Check sheet for the modelled part. Datum: model origin and axes. Units: mm. Face numbers are marked on the shaded views. A direction names the side the tool comes from. Round coordinates to 2 decimals unless told otherwise and drop trailing zeros. Loops run counter-clockwise (first coordinate to the right, second up) from the corner with the lowest first, then second, coordinate; pieces in that order, holes last. Notation, with made-up numbers: (63, -23) - (122, -23) arc R17 ccw to (122, 8) - close; hole circle Ø7 at (54.5, -32). An arc over 180 degrees is marked (long way). Put each result on its own line as item: value. Start each with the question number.
Item 1: Gauge pin test, flat ends, axial feed: pin 1 Ø8 at (x, y) = (-4, -1) entering from +Z; pin 2 Ø1 at (x, y) = (8, -2.5) entering from -Z. Record the tip position at first contact, or that the pin passes through.
Item 2: Draft check along Y on the marked faces 4, 5 and 6. Enter one of: pulls with the +Y half, pulls with the -Y half, needs draft (parallel to the pull), parting line crosses it, or undercut.
Item 3: Section check C-C, the plane z = 6.5. Record the cut outline in (x, y).
Item 4: Section check D-D, the plane y = 6. Record the cut outline in (x, z), and give its area (3 significant figures).
Item 5: Tool access check on the marked faces 1, 2 and 3. Record the directions out of +Z, -Z, +X, -X, +Y, -Y that give a thin tool (end or side, any length) a straight path to the whole face; none if there is none.
Item 6: Material ranges on line 1 along X through (y, z) = (0.5, 3); line 2 along Y through (x, z) = (6.5, 4); line 3 along Y through (x, z) = (4, 10.25), recorded low to high.
Item 7: Section check B-B, the plane x = -4. Record the cut outline in (y, z).
Item 8: Section check A-A, the plane z = 10.5. Record the cut outline in (x, y), and give its area (3 significant figures).
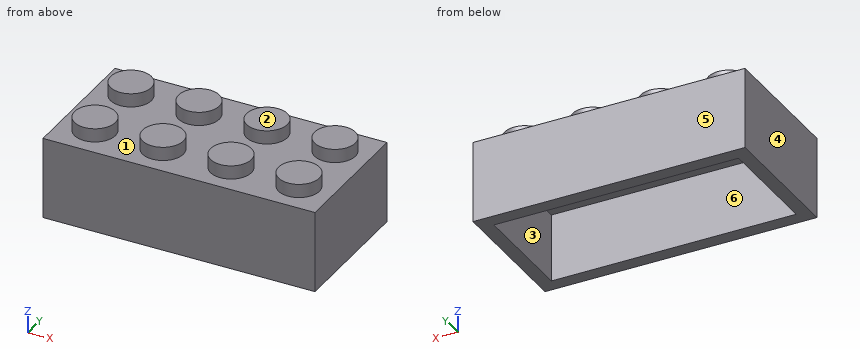
from build123d import *

# Parameters (mm, degrees)
F0_W     = 32
F0_H     = 16
F1_DEPTH = 9.6
F2_W     = 28.8
F2_H     = 12.8
F3_DEPTH = 8
F4_R     = 2.4
F5_DEPTH = 1.6


with BuildPart() as f1:
    # F0 (on Top) → F1 (new body)
    with BuildSketch(Plane.XY):
        Rectangle(F0_W, F0_H)
    extrude(amount=F1_DEPTH)

    # F2 (on face) → F3 (cut)
    with BuildSketch(Plane(origin=(0, 0, 0), x_dir=(1, 0, 0), z_dir=(0, 0, -1))):
        Rectangle(F2_W, F2_H)
    extrude(amount=-F3_DEPTH, mode=Mode.SUBTRACT)

    # F4 (on face) → F5 (join)
    with BuildSketch(Plane.XY.offset(9.6)):
        with Locations((-12, 4)):
            Circle(F4_R)
        with Locations((-4, 4)):
            Circle(F4_R)
        with Locations((4, 4)):
            Circle(F4_R)
        with Locations((12, 4)):
            Circle(F4_R)
        with Locations((-12, -4)):
            Circle(F4_R)
        with Locations((-4, -4)):
            Circle(F4_R)
        with Locations((4, -4)):
            Circle(F4_R)
        with Locations((12, -4)):
            Circle(F4_R)
    extrude(amount=F5_DEPTH)


solid = f1.part
Check result:
1. pin 1: z = 11.2
1. pin 2: z = 8
2. face 4: needs draft
2. face 5: pulls with the +Y half
2. face 6: undercut
3. outline: (-16, -8) - (16, -8) - (16, 8) - (-16, 8) - close; hole (-14.4, -6.4) - (14.4, -6.4) - (14.4, 6.4) - (-14.4, 6.4) - close
4. outline: (-16, 0) - (-14.4, 0) - (-14.4, 8) - (14.4, 8) - (14.4, 0) - (16, 0) - (16, 9.6) - (13.33, 9.6) - (13.33, 11.2) - (10.67, 11.2) - (10.67, 9.6) - (5.33, 9.6) - (5.33, 11.2) - (2.67, 11.2) - (2.67, 9.6) - (-2.67, 9.6) - (-2.67, 11.2) - (-5.33, 11.2) - (-5.33, 9.6) - (-10.67, 9.6) - (-10.67, 11.2) - (-13.33, 11.2) - (-13.33, 9.6) - (-16, 9.6) - close
4. area: 93.8 mm²
5. face 1: +Z
5. face 2: +Z, +X, -X, +Y, -Y
5. face 3: -Z
6. line 1: -16 to -14.4, 14.4 to 16
6. line 2: -8 to -6.4, 6.4 to 8
6. line 3: -6.4 to -1.6, 1.6 to 6.4
7. outline: (-8, 0) - (-6.4, 0) - (-6.4, 8) - (6.4, 8) - (6.4, 0) - (8, 0) - (8, 9.6) - (6.4, 9.6) - (6.4, 11.2) - (1.6, 11.2) - (1.6, 9.6) - (-1.6, 9.6) - (-1.6, 11.2) - (-6.4, 11.2) - (-6.4, 9.6) - (-8, 9.6) - close
8. outline: circle Ø4.8 at (-12, -4); circle Ø4.8 at (-12, 4); circle Ø4.8 at (-4, -4); circle Ø4.8 at (-4, 4); circle Ø4.8 at (4, -4); circle Ø4.8 at (4, 4); circle Ø4.8 at (12, -4); circle Ø4.8 at (12, 4)
8. area: 145 mm²
